Read the model definition and answer for the solid it produces. Units are mm, in the model's axes. A direction names the side the tool comes from. Give positions to 0.01 mm unless a question says otherwise; leave off trailing zeros. Write each loop counter-clockwise with the first axis right and the second up, starting at its lowest first coordinate (ties: lowest second). Pieces come first, ordered by that corner, then holes. Notation, with made-up numbers: M 43,67 L 73,67 A26 ccw 73,95 Z; hole C -24.75,14.5 d5. An arc over 180 degrees is marked long. Use a Markdown table: item, result. Add a question column.
Item 1: Consider probe 1 along Z at (x, y) = (-1, 25.25); probe 2 along Y at (x, z) = (0, -103.5) (3 decimals); probe 3 along Z at (x, y) = (13.25, 13.5). Determine where each line is inside the solid, lowest interval first. Write a range as [from, to].
Item 2: For faces 1 (the flat face through (16, 29, -35)), 2 (the flat face through (5, 15, 5)), 3 (the flat face through (-6, 15, -15)), determine the directions among +Z, -Z, +X, -X, +Y, -Y from which every point of the face is accessible in a straight line to the end or side of a thin tool.
Item 3: A cutting plane is placed at B-B on y = 22. Determine the outline of the cut face in (x, z).
Item 4: A cutting plane is placed at D-D on z = 2.5. Determine the outline of the cut face in (x, y) (3 decimals).
Item 5: The mould has two halves that part along Y. Classify faces 4 (the flat face through (6, 0, -49)), 5 (the flat face through (-5.05, 15, -95)), 6 (the flat face through (3, 15, 15)): pulls with the +Y half, pulls with the -Y half, needs draft (parallel to the pull), parting line crosses it, or undercut.
Item 6: Given P1, Ø1.5, axis at y = 2, z = -50, coming from the -X side; P2, Ø10, axis at x = 1.5, y = 11.5, coming from the -Z side; P3, Ø10, axis at y = 19, z = -102, coming from the +X side, each flat-ended and moving along its own axis, determine where each tip first touches the part or whether it passes through.
Item 7: A cutting plane is placed at C-C on x = 13.5. Determine the outline of the cut face in (y, z) (3 decimals), then the cut area to 3 significant figures.
Item 8: A cutting plane is placed at A-A on z = -55.5. Determine the outline of the cut face in (x, y) (3 decimals).
from build123d import *

# Parameters (mm, degrees)
SKETCH_1_W          = 30
SKETCH_1_H          = 30
EXTRUDE_1_DEPTH     = 30
SKETCH_2_W          = 20
SKETCH_2_H          = 20.05
CUT_EXTRUDE_1_DEPTH = 20
CUT_EXTRUDE_2_DEPTH = 20
SKETCH_4_W          = 5
SKETCH_4_H          = 30
CUT_EXTRUDE_3_DEPTH = 55
SKETCH_5_W          = 15
SKETCH_5_H          = 4.975
EXTRUDE_2_DEPTH     = 120
EXTRUDE_3_DEPTH     = 60
SKETCH_7_R          = 3.1
CUT_EXTRUDE_4_DEPTH = 60
CUT_EXTRUDE_5_REACH = 155.704
SKETCH_8_W          = 20.1
SKETCH_8_H          = 20.15
EXTRUDE_4_DEPTH     = 1
SKETCH_10_R         = 3.1
CUT_EXTRUDE_6_DEPTH = 10
SKETCH_12_W         = 26
SKETCH_12_H         = 20
CUT_EXTRUDE_8_DEPTH = 87


with BuildPart() as part:
    # 草图1 → 凸台-拉伸1 (new body)
    with BuildSketch(Plane(origin=(0, 0, 0), x_dir=(1, 0, 0), z_dir=(0, 1, 0))):
        Rectangle(SKETCH_1_W, SKETCH_1_H)
    extrude(amount=EXTRUDE_1_DEPTH)

    # 草图2 → 切除-拉伸1 (cut)
    with BuildSketch(Plane(origin=(15, 0, 0), x_dir=(0, 0, -1), z_dir=(1, 0, 0))):
        with Locations((5, 15)):
            Rectangle(SKETCH_2_W, SKETCH_2_H)
    extrude(amount=-CUT_EXTRUDE_1_DEPTH, mode=Mode.SUBTRACT)

    # 草图3 → 切除-拉伸2 (cut)
    with BuildSketch(Plane(origin=(-5, 0, 0), x_dir=(0, 0, -1), z_dir=(1, 0, 0))):
        with BuildLine():
            ThreePointArc((7.189292698, 17.194765929), (5, 18.1), (2.810707302, 17.194765929))
            Line((2.810707302, 17.194765929), (5, 15))
            Line((5, 15), (7.189292698, 17.194765929))
        make_face()
        with BuildLine():
            Line((5, 15), (2.810707302, 17.194765929))
            ThreePointArc((2.810707302, 17.194765929), (1.9, 15), (2.810707302, 12.805234071))
            Line((2.810707302, 12.805234071), (5, 15))
        make_face()
        with BuildLine():
            Line((7.189292698, 17.194765929), (5, 15))
            Line((5, 15), (7.189292698, 12.805234071))
            ThreePointArc((7.189292698, 12.805234071), (7.86328547, 13.81189381), (8.1, 15))
            ThreePointArc((8.1, 15), (7.86328547, 16.18810619), (7.189292698, 17.194765929))
        make_face()
        with BuildLine():
            Line((7.189292698, 12.805234071), (5, 15))
            Line((5, 15), (2.810707302, 12.805234071))
            ThreePointArc((2.810707302, 12.805234071), (5, 11.9), (7.189292698, 12.805234071))
        make_face()
        with BuildLine():
            ThreePointArc((7.189292698, 17.194765929), (5, 18.1), (2.810707302, 17.194765929))
            Line((2.810707302, 17.194765929), (5, 15))
            Line((5, 15), (7.189292698, 17.194765929))
        make_face()
        with BuildLine():
            Line((5, 15), (2.810707302, 17.194765929))
            ThreePointArc((2.810707302, 17.194765929), (1.9, 15), (2.810707302, 12.805234071))
            Line((2.810707302, 12.805234071), (5, 15))
        make_face()
        with BuildLine():
            Line((7.189292698, 17.194765929), (5, 15))
            Line((5, 15), (7.189292698, 12.805234071))
            ThreePointArc((7.189292698, 12.805234071), (7.86328547, 13.81189381), (8.1, 15))
            ThreePointArc((8.1, 15), (7.86328547, 16.18810619), (7.189292698, 17.194765929))
        make_face()
        with BuildLine():
            Line((7.189292698, 12.805234071), (5, 15))
            Line((5, 15), (2.810707302, 12.805234071))
            ThreePointArc((2.810707302, 12.805234071), (5, 11.9), (7.189292698, 12.805234071))
        make_face()
        with BuildLine():
            ThreePointArc((7.189292698, 17.194765929), (5, 18.1), (2.810707302, 17.194765929))
            Line((2.810707302, 17.194765929), (5, 15))
            Line((5, 15), (7.189292698, 17.194765929))
        make_face()
        with BuildLine():
            Line((5, 15), (2.810707302, 17.194765929))
            ThreePointArc((2.810707302, 17.194765929), (1.9, 15), (2.810707302, 12.805234071))
            Line((2.810707302, 12.805234071), (5, 15))
        make_face()
        with BuildLine():
            Line((7.189292698, 17.194765929), (5, 15))
            Line((5, 15), (7.189292698, 12.805234071))
            ThreePointArc((7.189292698, 12.805234071), (7.86328547, 13.81189381), (8.1, 15))
            ThreePointArc((8.1, 15), (7.86328547, 16.18810619), (7.189292698, 17.194765929))
        make_face()
        with BuildLine():
            Line((7.189292698, 12.805234071), (5, 15))
            Line((5, 15), (2.810707302, 12.805234071))
            ThreePointArc((2.810707302, 12.805234071), (5, 11.9), (7.189292698, 12.805234071))
        make_face()
        with BuildLine():
            ThreePointArc((7.189292698, 17.194765929), (5, 18.1), (2.810707302, 17.194765929))
            Line((2.810707302, 17.194765929), (5, 15))
            Line((5, 15), (7.189292698, 17.194765929))
        make_face()
        with BuildLine():
            Line((5, 15), (2.810707302, 17.194765929))
            ThreePointArc((2.810707302, 17.194765929), (1.9, 15), (2.810707302, 12.805234071))
            Line((2.810707302, 12.805234071), (5, 15))
        make_face()
        with BuildLine():
            Line((7.189292698, 17.194765929), (5, 15))
            Line((5, 15), (7.189292698, 12.805234071))
            ThreePointArc((7.189292698, 12.805234071), (7.86328547, 13.81189381), (8.1, 15))
            ThreePointArc((8.1, 15), (7.86328547, 16.18810619), (7.189292698, 17.194765929))
        make_face()
        with BuildLine():
            Line((7.189292698, 12.805234071), (5, 15))
            Line((5, 15), (2.810707302, 12.805234071))
            ThreePointArc((2.810707302, 12.805234071), (5, 11.9), (7.189292698, 12.805234071))
        make_face()
    extrude(amount=-CUT_EXTRUDE_2_DEPTH, mode=Mode.SUBTRACT)

    # 草图4 → 切除-拉伸3 (cut)
    with BuildSketch(Plane.XZ):
        with Locations((-12.5, 0)):
            Rectangle(SKETCH_4_W, SKETCH_4_H)
    extrude(amount=-CUT_EXTRUDE_3_DEPTH, mode=Mode.SUBTRACT)

    # 草图5 → 凸台-拉伸2 (add)
    with BuildSketch(Plane(origin=(0, 0, -15), x_dir=(-1, 0, 0), z_dir=(0, 0, -1))):
        with Locations((-7.5, 27.5125)):
            Rectangle(SKETCH_5_W, SKETCH_5_H)
        with Locations((-7.5, 2.4875)):
            Rectangle(SKETCH_5_W, SKETCH_5_H)
    extrude(amount=EXTRUDE_2_DEPTH)

    # 草图6 → 凸台-拉伸3 (add)
    with BuildSketch(Plane(origin=(0, 0, -135), x_dir=(-1, 0, 0), z_dir=(0, 0, -1))):
        Polygon((5, 4.975), (0, 4.975), (0, 0), (10, 0), (10, 30), (0, 30), (0, 25.025), (5, 25.025), align=None)
    extrude(amount=-EXTRUDE_3_DEPTH)

    # 草图7 → 切除-拉伸4 (cut)
    with BuildSketch(Plane.ZY.offset(10)):
        with Locations((-85, 15)):
            Circle(SKETCH_7_R)
    extrude(amount=-CUT_EXTRUDE_4_DEPTH, mode=Mode.SUBTRACT)

    # 切除-拉伸5: up to this face of the body (flat: up to its plane)
    cut_extrude_5_end = Plane(part.part.faces().sort_by_distance((5, 15, 5))[0])
    # 草图8 → 切除-拉伸5 (cut, up to the picked face)
    with BuildSketch(Plane(origin=(0, 0, -135), x_dir=(-1, 0, 0), z_dir=(0, 0, -1)), mode=Mode.PRIVATE) as cut_extrude_5_sk1:
        with Locations((-5, 15)):
            Rectangle(SKETCH_8_W, SKETCH_8_H)
    cut_extrude_5_tool1 = split(extrude(cut_extrude_5_sk1.sketch, amount=-CUT_EXTRUDE_5_REACH, mode=Mode.PRIVATE), bisect_by=cut_extrude_5_end, keep=Keep.BOTH, mode=Mode.PRIVATE)
    add(cut_extrude_5_tool1.solids().sort_by(Axis((5, 15, -135), (0, 0, 1)))[0], mode=Mode.SUBTRACT)

    # 草图9 → 凸台-拉伸4 (add)
    with BuildSketch(Plane(origin=(15, 0, 0), x_dir=(0, 0, -1), z_dir=(1, 0, 0))):
        Polygon((135, 4.925), (-5, 4.925), (-5, 25.075), (135, 25.075), (135, 30), (-15, 30), (-15, 0), (135, 0), align=None)
    extrude(amount=EXTRUDE_4_DEPTH)

    # 草图10 → 切除-拉伸6 (cut)
    # profile 1 of 9: a face of its own
    with BuildSketch(Plane.ZY.offset(10)):
        with BuildLine():
            ThreePointArc((-99.75, 15), (-99.948207558, 16.428948256), (-100.527864045, 17.75))
            ThreePointArc((-100.527864045, 17.75), (-101.830321577, 19.185168897), (-103.564729991, 20.05))
            Line((-103.564729991, 20.05), (-106.435270009, 20.05))
            ThreePointArc((-106.435270009, 20.05), (-108.169678423, 19.185168897), (-109.472135955, 17.75))
            ThreePointArc((-109.472135955, 17.75), (-110.25, 15), (-109.472135955, 12.25))
            ThreePointArc((-109.472135955, 12.25), (-108.169678423, 10.814831103), (-106.435270009, 9.95))
            Line((-106.435270009, 9.95), (-103.564729991, 9.95))
            ThreePointArc((-103.564729991, 9.95), (-101.830321577, 10.814831103), (-100.527864045, 12.25))
            ThreePointArc((-100.527864045, 12.25), (-99.948207558, 13.571051744), (-99.75, 15))
        make_face()
    # profile 2 of 9: a face of its own
    with BuildSketch(Plane.ZY.offset(10)):
        with BuildLine():
            Line((-106.435270009, 20.05), (-103.564729991, 20.05))
            ThreePointArc((-103.564729991, 20.05), (-105, 20.25), (-106.435270009, 20.05))
        make_face()
    # profile 3 of 9: a face of its own
    with BuildSketch(Plane.ZY.offset(10)):
        with BuildLine():
            ThreePointArc((-106.435270009, 9.95), (-105, 9.75), (-103.564729991, 9.95))
            Line((-103.564729991, 9.95), (-106.435270009, 9.95))
        make_face()
    # profile 4 of 9: a face of its own
    with BuildSketch(Plane.ZY.offset(10)):
        with BuildLine():
            ThreePointArc((-79.75, 15), (-79.948207558, 16.428948256), (-80.527864045, 17.75))
            ThreePointArc((-80.527864045, 17.75), (-81.830321577, 19.185168897), (-83.564729991, 20.05))
            Line((-83.564729991, 20.05), (-86.435270009, 20.05))
            ThreePointArc((-86.435270009, 20.05), (-88.169678423, 19.185168897), (-89.472135955, 17.75))
            ThreePointArc((-89.472135955, 17.75), (-90.25, 15), (-89.472135955, 12.25))
            ThreePointArc((-89.472135955, 12.25), (-88.169678423, 10.814831103), (-86.435270009, 9.95))
            Line((-86.435270009, 9.95), (-83.564729991, 9.95))
            ThreePointArc((-83.564729991, 9.95), (-81.830321577, 10.814831103), (-80.527864045, 12.25))
            ThreePointArc((-80.527864045, 12.25), (-79.948207558, 13.571051744), (-79.75, 15))
        make_face()
        with Locations((-85, 15)):
            Circle(SKETCH_10_R, mode=Mode.SUBTRACT)
    # profile 5 of 9: a face of its own
    with BuildSketch(Plane.ZY.offset(10)):
        with BuildLine():
            Line((-86.435270009, 20.05), (-83.564729991, 20.05))
            ThreePointArc((-83.564729991, 20.05), (-85, 20.25), (-86.435270009, 20.05))
        make_face()
    # profile 6 of 9: a face of its own
    with BuildSketch(Plane.ZY.offset(10)):
        with BuildLine():
            ThreePointArc((-86.435270009, 9.95), (-85, 9.75), (-83.564729991, 9.95))
            Line((-83.564729991, 9.95), (-86.435270009, 9.95))
        make_face()
    # profile 7 of 9: a face of its own
    with BuildSketch(Plane.ZY.offset(10)):
        with BuildLine():
            ThreePointArc((0.25, 15), (0.051792442, 16.428948256), (-0.527864045, 17.75))
            ThreePointArc((-0.527864045, 17.75), (-1.830321577, 19.185168897), (-3.564729991, 20.05))
            Line((-3.564729991, 20.05), (-6.435270009, 20.05))
            ThreePointArc((-6.435270009, 20.05), (-8.169678423, 19.185168897), (-9.472135955, 17.75))
            ThreePointArc((-9.472135955, 17.75), (-10.25, 15), (-9.472135955, 12.25))
            ThreePointArc((-9.472135955, 12.25), (-8.169678423, 10.814831103), (-6.435270009, 9.95))
            Line((-6.435270009, 9.95), (-3.564729991, 9.95))
            ThreePointArc((-3.564729991, 9.95), (-1.830321577, 10.814831103), (-0.527864045, 12.25))
            ThreePointArc((-0.527864045, 12.25), (0.051792442, 13.571051744), (0.25, 15))
        make_face()
    # profile 8 of 9: a face of its own
    with BuildSketch(Plane.ZY.offset(10)):
        with BuildLine():
            Line((-6.435270009, 20.05), (-3.564729991, 20.05))
            ThreePointArc((-3.564729991, 20.05), (-5, 20.25), (-6.435270009, 20.05))
        make_face()
    # profile 9 of 9: a face of its own
    with BuildSketch(Plane.ZY.offset(10)):
        with BuildLine():
            ThreePointArc((-6.435270009, 9.95), (-5, 9.75), (-3.564729991, 9.95))
            Line((-3.564729991, 9.95), (-6.435270009, 9.95))
        make_face()
    extrude(amount=-CUT_EXTRUDE_6_DEPTH, mode=Mode.SUBTRACT)

    # 草图12 → 切除-拉伸8 (cut)
    with BuildSketch(Plane.XZ):
        with Locations((3, -125)):
            Rectangle(SKETCH_12_W, SKETCH_12_H)
    extrude(amount=-CUT_EXTRUDE_8_DEPTH, mode=Mode.SUBTRACT)


solid = part.part
Filled in:
| question | item | result |
|---|---|---|
| 1 | probe 1 | [-115, -75], [-15, 15] |
| 1 | probe 2 | [0, 4.925], [25.075, 30] |
| 1 | probe 3 | [5, 15] |
| 2 | face 1 | +Z, -Z, +X, +Y, -Y |
| 2 | face 2 | -Z, +X |
| 2 | face 3 | -X, +Y, -Y |
| 3 | outline | M -10,-115 L -5.05,-115 L -5.05,-75 L -10,-75 Z; M -10,-15 L -5.05,-15 L -5.05,5 L 16,5 L 16,15 L -10,15 Z |
| 4 | outline | M -10,0 L 16,0 L 16,4.925 L -5.05,4.925 L -5.05,25.075 L 16,25.075 L 16,30 L -10,30 Z |
| 5 | face 4 | pulls with the -Y half |
| 5 | face 5 | undercut |
| 5 | face 6 | needs draft |
| 6 | P1 | x = 0 |
| 6 | P2 | z = 5 |
| 6 | P3 | x = -5.05 |
| 7 | outline | M 0,-115 L 4.925,-115 L 4.925,5 L 25.075,5 L 25.075,-115 L 30,-115 L 30,15 L 0,15 Z |
| 7 | area | 1,480 mm² |
| 8 | outline | M 0,0 L 16,0 L 16,4.925 L 0,4.925 Z; M 0,25.075 L 16,25.075 L 16,30 L 0,30 Z |
